Can you work these out from the drawing? Everything is in mm from the part's minimum corner. Coordinates: 2 decimals unless noted, no trailing zeros. Loops run counter-clockwise (first coordinate to the right, second up) from the corner with the lowest first, then second, coordinate; pieces in that order, holes last. Notation, with made-up numbers: M 72,53 L 116,53 A22 cw 116,64 Z; hole C 30,-1 d3. An arc over 180 degrees is marked long. Use CSV: the item, a comma, the result in double quotes. Start each with the question number.
Q1. If we section it at C-C (x = 72.5): Please give me the cut outline in (y, z), and give its area (3 significant figures).
Q2. If we section it at B-B (z = 128): Please give me the cut outline in (x, y).
Q3. Please list where these lines run through material, in increasing order: probe 1 along X at (y, z) = (1.35, 79); probe 2 along Z at (x, y) = (127, 2.4). Write a range as [from, to].
Q4. If we section it at A-A (y = 3.6): Please give me the cut outline in (x, z).
Q5. For pin 1 Ø1.7 at (x, y) = (2, 4) entering from -Z; pin 2 Ø1.5 at (x, z) = (41.5, 75) entering from -Y; pin 3 Ø3 at (y, z) = (2, 14.5) entering from +X; pin 4 Ø1.7 at (x, y) = (20, 4) entering from -Z, each with a flat end and sliding along its axis, tell me the tip position at first contact or that it passes through.
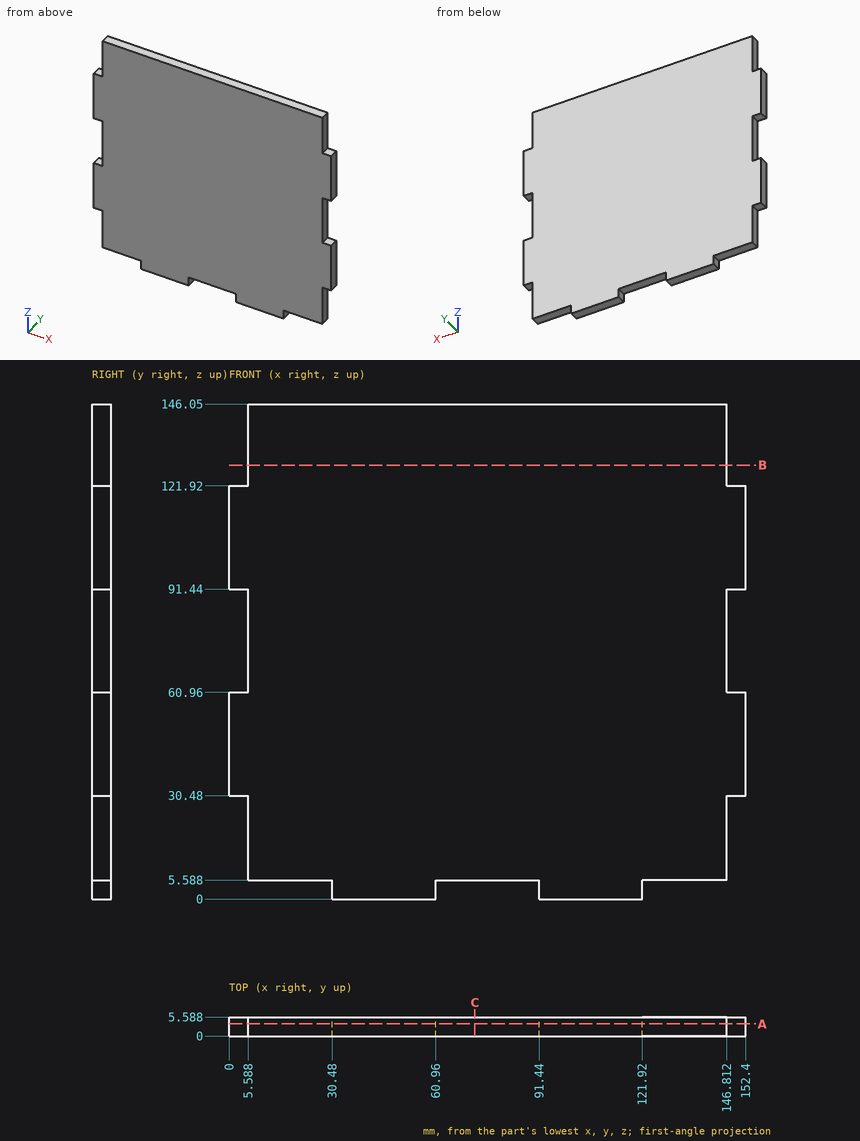
Results below:
1,outline,"M 0,5.59 L 5.59,5.59 L 5.59,146.05 L 0,146.05 Z"
1,area,"785 mm^2"
2,outline,"M 5.59,0 L 146.81,0 L 146.81,5.59 L 5.59,5.59 Z"
3,probe 1,"[5.59, 146.81]"
3,probe 2,"[5.59, 146.05]"
4,outline,"M 0,30.48 L 5.59,30.48 L 5.59,5.59 L 30.48,5.59 L 30.48,0 L 60.96,0 L 60.96,5.59 L 91.44,5.59 L 91.44,0 L 121.92,0 L 121.92,5.59 L 146.81,5.59 L 146.81,30.48 L 152.4,30.48 L 152.4,60.96 L 146.81,60.96 L 146.81,91.44 L 152.4,91.44 L 152.4,121.92 L 146.81,121.92 L 146.81,146.05 L 5.59,146.05 L 5.59,121.92 L 0,121.92 L 0,91.44 L 5.59,91.44 L 5.59,60.96 L 0,60.96 Z"
5,pin 1,"z = 30.48"
5,pin 2,"y = 0"
5,pin 3,"x = 146.81"
5,pin 4,"z = 5.59"
